Here's the drawing with two shaded views (mm, measured from the low corner). I have some questions. Coordinates: 2 decimals unless noted, no trailing zeros. Write each loop counter-clockwise with the first axis right and the second up, starting at its lowest first coordinate (ties: lowest second). Pieces come first, ordered by that corner, then holes.
Item 1: I'm going to push flat-ended pins straight in: pin 1 Ø10 at (y, z) = (129.5, 8.5) entering from +X; pin 2 Ø3.5 at (x, y) = (18, 19.5) entering from +Z (1 decimal); pin 3 Ø2.5 at (x, y) = (18.5, 21) entering from -Z; pin 4 Ø6.5 at (y, z) = (16, 10.5) entering from +X. Where does each tip first touch, or does it pass through?
Item 2: If we section it at A-A (y = 118.5): Please give me the cut outline in (x, z).
Item 3: If we section it at C-C (z = 16.75): Please give me the cut outline in (x, y).
Item 4: If we section it at B-B (x = 5): Please give me the cut outline in (y, z).
Item 5: If I drill on line 1 (Z direction, x = 10, y = 57); line 2 (X direction, y = 73.5, z = 9.5); line 3 (X direction, y = 16.5, z = 8), over which ranges is the centre line in solid material (lowest first)?
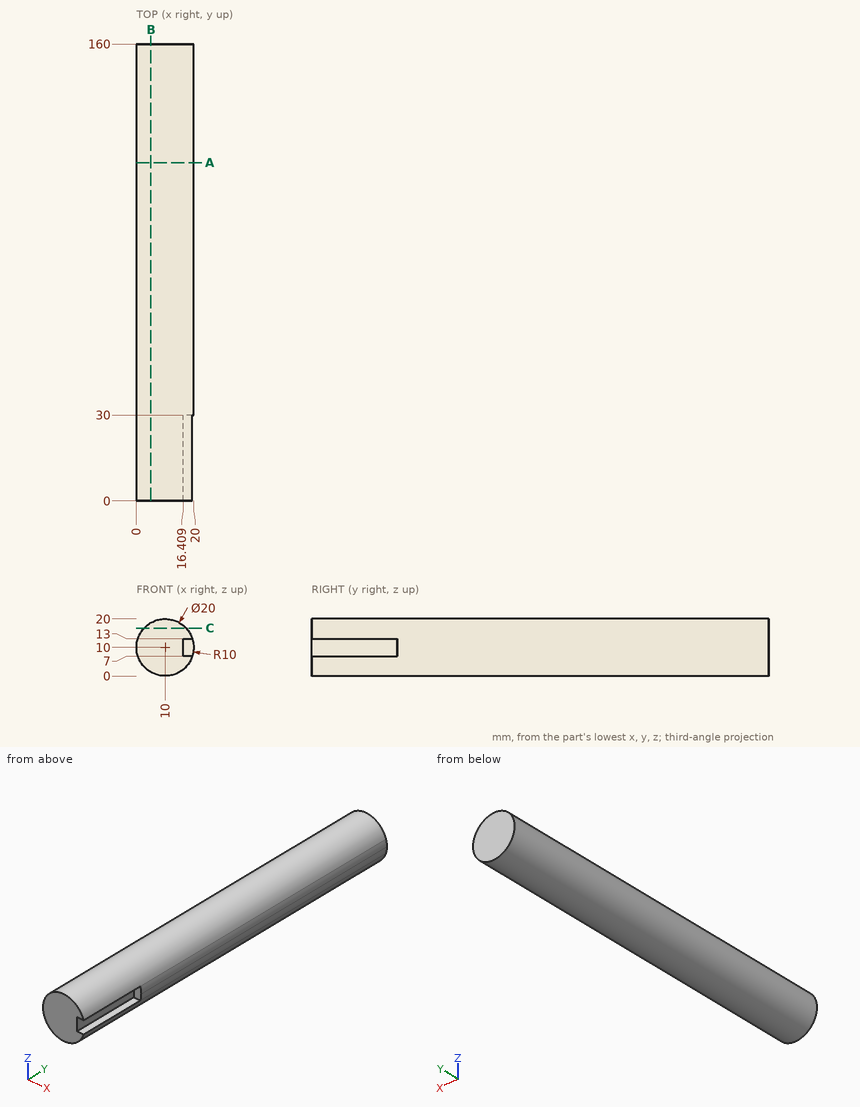
Answer list:
1. pin 1: stops at x = 20
1. pin 2: stops at z = 17.8
1. pin 3: stops at z = 3.11
1. pin 4: stops at x = 19.54
2. outline: circle Ø20 at (10, 10)
3. outline: (2.62, 0) - (17.38, 0) - (17.38, 160) - (2.62, 160) - close
4. outline: (0, 1.34) - (160, 1.34) - (160, 18.66) - (0, 18.66) - close
5. line 1: z = 0 to 20
5. line 2: x = 0.01 to 19.99
5. line 3: x = 0.2 to 16.41
